from build123d import *

# Parameters (mm, degrees)
BOSS_EXTRUDE1_DEPTH = 50.8
SKETCH3_R           = 3.3782
CUT_EXTRUDE1_DEPTH  = 25.4
SKETCH4_R           = 3.3782
CUT_EXTRUDE2_DEPTH  = 25.4
SKETCH7_W           = 228.6
SKETCH7_H           = 152.4
CUT_EXTRUDE5_DEPTH  = 19.05
SKETCH8_W           = 228.6
SKETCH8_H           = 25.4
CUT_EXTRUDE6_DEPTH  = 39.37
SKETCH9_R           = 3.3782
CUT_EXTRUDE7_DEPTH  = 27.94
CUT_EXTRUDE8_DEPTH  = 40.64
SKETCH12_W          = 1.27
SKETCH12_H          = 31.75
CUT_EXTRUDE9_DEPTH  = 16.51
CUT_EXTRUDE10_REACH = 33.75
SKETCH13_R          = 3.3782


with BuildPart() as part:
    # Sketch2 → Boss-Extrude1 (new body)
    with BuildSketch(Plane.XY):
        with BuildLine():
            Line((215.9, 0), (228.6, 0))
            Line((228.6, 0), (228.6, 101.6))
            Line((228.6, 101.6), (174.752, 152.4))
            Line((174.752, 152.4), (156.972, 152.4))
            ThreePointArc((156.972, 152.4), (143.51, 138.938), (130.048, 152.4))
            Line((130.048, 152.4), (98.552, 152.4))
            ThreePointArc((98.552, 152.4), (85.09, 138.938), (71.628, 152.4))
            Line((71.628, 152.4), (53.848, 152.4))
            Line((53.848, 152.4), (0, 101.6))
            Line((0, 101.6), (0, 0))
            Line((0, 0), (12.7, 0))
            Line((12.7, 0), (12.7, 76.2))
            Line((12.7, 76.2), (215.9, 76.2))
            Line((215.9, 76.2), (215.9, 0))
        make_face()
    extrude(amount=BOSS_EXTRUDE1_DEPTH)

    # Sketch3 → Cut-Extrude1 (cut)
    with BuildSketch(Plane.ZY):
        with Locations((25.4, 63.5)):
            Circle(SKETCH3_R)
        with Locations((25.4, 38.1)):
            Circle(SKETCH3_R)
    extrude(amount=-CUT_EXTRUDE1_DEPTH, mode=Mode.SUBTRACT)

    # Sketch4 → Cut-Extrude2 (cut)
    with BuildSketch(Plane(origin=(228.6, 0, 0), x_dir=(0, 0, -1), z_dir=(1, 0, 0))):
        with Locations((-25.4, 63.5)):
            Circle(SKETCH4_R)
        with Locations((-25.4, 38.1)):
            Circle(SKETCH4_R)
    extrude(amount=-CUT_EXTRUDE2_DEPTH, mode=Mode.SUBTRACT)

    # Sketch7 → Cut-Extrude5 (cut)
    with BuildSketch(Plane.XY.offset(50.8)):
        with Locations((114.3, 76.2)):
            Rectangle(SKETCH7_W, SKETCH7_H)
    extrude(amount=-CUT_EXTRUDE5_DEPTH, mode=Mode.SUBTRACT)

    # Sketch8 → Cut-Extrude6 (cut)
    with BuildSketch(Plane.XY.offset(31.75)):
        with Locations((114.3, 12.7)):
            Rectangle(SKETCH8_W, SKETCH8_H)
    extrude(amount=-CUT_EXTRUDE6_DEPTH, mode=Mode.SUBTRACT)

    # Sketch9 → Cut-Extrude7 (cut)
    with BuildSketch(Plane(origin=(0, 152.4, 0), x_dir=(1, 0, 0), z_dir=(0, 1, 0))):
        with Locations((60.198, -15.875)):
            Circle(SKETCH9_R)
        with Locations((114.3, -15.875)):
            Circle(SKETCH9_R)
        with Locations((168.402, -15.875)):
            Circle(SKETCH9_R)
    extrude(amount=-CUT_EXTRUDE7_DEPTH, mode=Mode.SUBTRACT)

    # Sketch10 → Cut-Extrude8 (cut)
    with BuildSketch(Plane.XY.offset(31.75)):
        Polygon((27.760759157, 101.6), (54.684759157, 127), (173.915240843, 127), (200.839240843, 101.6), align=None)
    extrude(amount=-CUT_EXTRUDE8_DEPTH, mode=Mode.SUBTRACT)

    # Sketch12 → Cut-Extrude9 (cut)
    with BuildSketch(Plane(origin=(0, 152.4, 0), x_dir=(1, 0, 0), z_dir=(0, 1, 0))):
        with Locations((85.725, -15.875)):
            Rectangle(SKETCH12_W, SKETCH12_H)
        with Locations((84.455, -15.875)):
            Rectangle(SKETCH12_W, SKETCH12_H)
        Polygon((143.51, 0), (142.24, 0), (142.24, -31.75), (144.78, -31.75), (144.78, 0), align=None)
    extrude(amount=-CUT_EXTRUDE9_DEPTH, mode=Mode.SUBTRACT)

    # Sketch13 → Cut-Extrude10 (cut, up to next)
    with BuildSketch(Plane.XY.offset(31.75), mode=Mode.PRIVATE) as cut_extrude10_sk1:
        with Locations((48.768, 95.25)):
            Circle(SKETCH13_R)
    cut_extrude10_tool1 = extrude(cut_extrude10_sk1.sketch, amount=-CUT_EXTRUDE10_REACH, mode=Mode.PRIVATE) & part.part
    add(cut_extrude10_tool1.solids().sort_by_distance((48.768, 95.25, 31.75))[0], mode=Mode.SUBTRACT)
    # Sketch13 → Cut-Extrude10 (cut, up to next)
    with BuildSketch(Plane.XY.offset(31.75), mode=Mode.PRIVATE) as cut_extrude10_sk2:
        with Locations((185.674, 95.25)):
            Circle(SKETCH13_R)
    cut_extrude10_tool2 = extrude(cut_extrude10_sk2.sketch, amount=-CUT_EXTRUDE10_REACH, mode=Mode.PRIVATE) & part.part
    add(cut_extrude10_tool2.solids().sort_by_distance((185.674, 95.25, 31.75))[0], mode=Mode.SUBTRACT)


solid = part.part
Source: CAD feature listing. Evaluate the final solid. Frame: model axes, mm. A direction names the side the tool comes from. Round coordinates to 2 decimals unless told otherwise and drop trailing zeros. Order: outer loops, then holes, each group sorted by start corner. A loop starts at its lowest first (then second) coordinate and runs counter-clockwise, first axis right, second up. Notation, with made-up numbers: (35.5, 52) - (59.5, 52) arc R22 cw to (59.5, 59) - close; hole circle Ø5 at (16, -33). An arc over 180 degrees is marked (long way). Use a Markdown table: item, result. Add a question column.
1. Section query C-C (y = 95.25). Return the cut outline in (x, z), then the cut area to 3 significant figures.
2. Section query B-B (x = 68.5). Return the cut outline in (y, z).
3. Section query A-A (y = 44.5). Return the cut outline in (x, z).
4. Set-up query: faces 1 (the flat face through (113, 76.2, 16)), 2 (the flat face through (113, 127, 20)), 3 (the cylindrical face through (117.522, 139.878, 14.86)). Return all of +Z, -Z, +X, -X, +Y, -Y with unobstructed straight access to the full face (end or side cutting, diameter ignored); none if empty.
5. Mould query, pull axis Y, two halves, no side actions, for faces 4 (the cylindrical face through (222.34, 60.2, 26.13)), 5 (the flat face through (164, 152.4, 16)), 6 (the cylindrical face through (165.912, 139.878, 13.592)). Classes: +Y half, -Y half, draft (parallel to the pull), parting line (faces both ways), or undercut.
6. First-contact query: pin 1 (2.5 mm diameter, centred on y = 136.5, z = 10.5, fed in from +X); pin 2 (8 mm diameter, centred on y = 135.5, z = 25.5, fed in from +X); pin 3 (4 mm diameter, centred on y = 122, z = 26, fed in from +X); pin 4 (8 mm diameter, centred on x = 60.198, z = 15.875, fed in from +Y). Flat tips, straight axial feed; report the tip coordinate or a pass-through.
7. Section query D-D (z = 4). Return the cut outline in (x, y).
8. Line query: probe 1 along Z at (x, y) = (114.3, 140); probe 2 along X at (y, z) = (50, 13); probe 3 along X at (y, z) = (147.5, 23). Output: solid intervals per line, ascending.
Derived:
| question | item | result |
|---|---|---|
| 1 | outline | (0, 0) - (45.39, 0) - (45.39, 31.75) - (0, 31.75) - close; (52.15, 0) - (182.3, 0) - (182.3, 31.75) - (52.15, 31.75) - close; (189.05, 0) - (228.6, 0) - (228.6, 31.75) - (189.05, 31.75) - close |
| 1 | area | 6,830 mm2 |
| 2 | outline | (76.2, 0) - (101.6, 0) - (101.6, 31.75) - (76.2, 31.75) - close; (127, 0) - (152.4, 0) - (152.4, 31.75) - (127, 31.75) - close |
| 3 | outline | (0, 0) - (12.7, 0) - (12.7, 31.75) - (0, 31.75) - close; (215.9, 0) - (228.6, 0) - (228.6, 31.75) - (215.9, 31.75) - close |
| 4 | face 1 | +Z, -Z, -Y |
| 4 | face 2 | +Z, -Z |
| 4 | face 3 | +Y |
| 5 | face 4 | undercut |
| 5 | face 5 | +Y half |
| 5 | face 6 | draft |
| 6 | pin 1 | x = 192.93 |
| 6 | pin 2 | x = 196.91 |
| 6 | pin 3 | x = 209.1 |
| 6 | pin 4 | y = 152.4 |
| 7 | outline | (0, 25.4) - (12.7, 25.4) - (12.7, 76.2) - (215.9, 76.2) - (215.9, 25.4) - (228.6, 25.4) - (228.6, 101.6) - (174.75, 152.4) - (156.97, 152.4) arc R13.46 cw to (144.78, 139) - (144.78, 135.89) - (142.24, 135.89) - (142.24, 139) arc R13.46 cw to (130.05, 152.4) - (98.55, 152.4) arc R13.46 cw to (86.36, 139) - (86.36, 135.89) - (83.82, 135.89) - (83.82, 139) arc R13.46 cw to (71.63, 152.4) - (53.85, 152.4) - (0, 101.6) - close; hole (27.76, 101.6) - (200.84, 101.6) - (173.92, 127) - (54.68, 127) - close; hole circle Ø6.76 at (48.77, 95.25); hole circle Ø6.76 at (185.67, 95.25) |
| 8 | probe 1 | 0 to 12.5, 19.25 to 31.75 |
| 8 | probe 2 | 0 to 12.7, 215.9 to 228.6 |
| 8 | probe 3 | 48.65 to 72.55, 97.63 to 130.97, 156.05 to 179.95 |
